from build123d import *

# Parameters (mm, degrees)
CYLINDER001_R               = 15
CYLINDER001_DEPTH           = 30
CYLINDER001_ROLL_ANGLE      = 57.515834
CYLINDER001_PITCH_ANGLE     = -33.522488
CYLINDER001_PLACEMENT_ANGLE = 57.515834
CYLINDER_R                  = 15
CYLINDER_DEPTH              = 30
SKETCH_W                    = 243.943557
SKETCH_H                    = 232.19397
SKETCH_R                    = 16.531402
SKETCH_W_2                  = 64.902409
SKETCH_H_2                  = 49.795826
PAD_DEPTH                   = 30
POCKET_DEPTH                = 10


with BuildPart() as cylinder001:
    # Cylinder001 → Cylinder001 (new body)
    with BuildSketch(Plane.XY):
        Circle(CYLINDER001_R)
    extrude(amount=CYLINDER001_DEPTH)


with BuildPart() as cylinder001_1:
    # Cylinder001 roll: moved
    add(cylinder001.part.rotate(Axis((0, 0, 0), (1, 0, 0)), CYLINDER001_ROLL_ANGLE))


with BuildPart() as cylinder001_2:
    # Cylinder001 pitch: moved
    add(cylinder001_1.part.rotate(Axis((0, 0, 0), (0, 1, 0)), CYLINDER001_PITCH_ANGLE))


with BuildPart() as cylinder001_3:
    # Cylinder001 placement: moved
    add(cylinder001_2.part.moved(Location((74, 69, 27))).rotate(Axis((74, 69, 27), (0, 0, 1)), CYLINDER001_PLACEMENT_ANGLE))


with BuildPart() as cylinder:
    # Cylinder → Cylinder (new body)
    with BuildSketch(Plane(origin=(74, 15, 31), x_dir=(1, 0, 0), z_dir=(0, -1, 0))):
        Circle(CYLINDER_R)
    extrude(amount=CYLINDER_DEPTH)


with BuildPart() as sphere:
    # Sphere → Sphere (revolve)
    with BuildSketch(Plane(origin=(0, 0, 38), x_dir=(1, 0, 0), z_dir=(0, -1, 0))):
        with BuildLine():
            ThreePointArc((0, -25), (25, 0), (0, 25))
            Line((0, 25), (0, -25))
        make_face()
    revolve(axis=Axis((0, 0, 38), (0, 0, 1)))


with BuildPart() as cut002:
    # Sketch → Pad (new body)
    with BuildSketch(Plane.XY):
        with Locations((4.089295, -7.505798)):
            Rectangle(SKETCH_W, SKETCH_H)
        with Locations((21.433901, -86.675552)):
            Circle(SKETCH_R, mode=Mode.SUBTRACT)
        with Locations((-55.777578, -84.157782)):
            Rectangle(SKETCH_W_2, SKETCH_H_2, mode=Mode.SUBTRACT)
    extrude(amount=PAD_DEPTH)

    # Sketch001 (on Face11 of Pad) → Pocket (cut)
    with BuildSketch(Plane.XY.offset(30)):
        Polygon((-80.299553, -22.364969), (-80.304949, -5.533931), (-94.883753, 2.876915), (-109.457161, -5.543277), (-109.451765, -22.374315), (-94.872961, -30.785161), align=None)
        with BuildLine():
            add(Edge.make_bspline(
                [(100.814049, -81.240913), (126.605952, -57.691792), (78.384447, -30.776448), (30.162942, -3.861103), (52.592544, -54.325568), (75.022146, -104.790034), (100.814049, -81.240913)],
                knots=[0, 0, 0, 2.094395, 2.094395, 4.18879, 4.18879, 6.283185, 6.283185, 6.283185], degree=2, weights=[1, 0.5, 1, 0.5, 1, 0.5, 1]))
        make_face()
    extrude(amount=-POCKET_DEPTH, mode=Mode.SUBTRACT)

    # Cut: cut Sphere
    add(sphere.part, mode=Mode.SUBTRACT)

    # Cut001: cut Cylinder
    add(cylinder.part, mode=Mode.SUBTRACT)

    # Cut002: cut Cylinder001
    add(cylinder001_3.part, mode=Mode.SUBTRACT)


solid = cut002.part
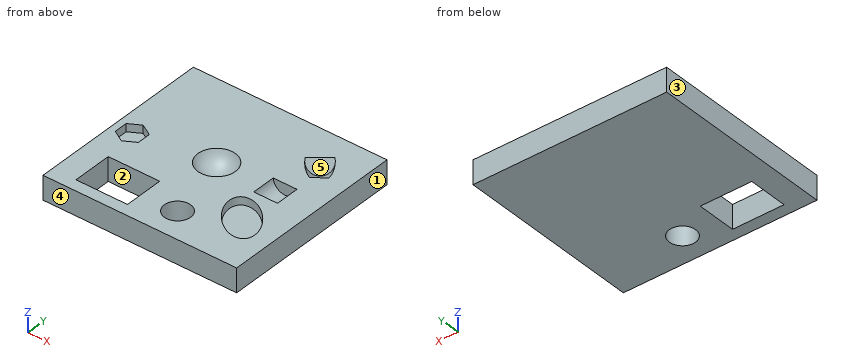
Geometry: final body of the model. Coordinates: model frame, mm. Face numbers are marked on the shaded views. A direction names the side the tool comes from. Round coordinates to 2 decimals unless told otherwise and drop trailing zeros. Order: outer loops, then holes, each group sorted by start corner. A loop starts at its lowest first (then second) coordinate and runs counter-clockwise, first axis right, second up. Notation, with made-up numbers: (80, 42) -> (86, 42) arc R13 cw to (86, 49) -> close; hole circle Ø5 at (83.25, 27.5). An arc over 180 degrees is marked (long way). Put each result on its own line as item: value. Start each with the question number.
Q1. First-contact query: pin 1 (8.5 mm diameter, centred on x = -101, y = -13, fed in from +Z). Flat tip, straight axial feed; report the tip coordinate or a pass-through.
Q2. Section B-B on z = 8. Return the cut outline in (x, y), and give its area (3 significant figures).
Q3. Section C-C on y = -18. Return the cut outline in (x, z).
Q4. Line query: probe 1 along X at (y, z) = (-99, 11.5); probe 2 along Y at (x, z) = (-72, 9); probe 3 along Z at (x, y) = (98, -76.5). Output: solid intervals per line, ascending.
Q5. Pull-direction query (Y, two-part tool) for the marked faces 3, 4 and 5; classes: +Y half, -Y half, draft (parallel to the pull), parting line (faces both ways), or undercut.
Q6. Reachability of the marked faces 1 and 2 from +Z, -Z, +X, -X, +Y, -Y: full face, straight path, thin tool, end or side. Return the list, or none.
Q7. Section A-A on x = -34. Return the cut outline in (y, z).
Ans:
1. pin 1: stops at z = 20
2. outline: (-117.88, -123.6) -> (126.06, -123.6) -> (126.06, 108.59) -> (-117.88, 108.59) -> close; hole (-88.23, -109.06) -> (-23.33, -109.06) -> (-23.33, -59.26) -> (-88.23, -59.26) -> close; hole circle Ø33.06 at (21.43, -86.68)
2. area: 52,600 mm2
3. outline: (-117.88, 0) -> (126.06, 0) -> (126.06, 30) -> (15.39, 30) arc R17.35 cw to (-15.39, 30) -> (-80.3, 30) -> (-80.3, 20) -> (-109.45, 20) -> (-109.45, 30) -> (-117.88, 30) -> close
4. probe 1: x = -117.88 to -88.23, -23.33 to 10.42, 32.45 to 126.06
4. probe 2: y = -123.6 to -109.06, -59.26 to 108.59
4. probe 3: z = 0 to 20
5. face 3: draft
5. face 4: -Y half
5. face 5: undercut
6. face 1: +Z, -Z, +X, +Y, -Y
6. face 2: +Z, -Z
7. outline: (-123.6, 0) -> (-109.06, 0) -> (-109.06, 30) -> (-123.6, 30) -> close; (-59.26, 0) -> (108.59, 0) -> (108.59, 30) -> (-59.26, 30) -> close
